from build123d import *

# Parameters (mm, degrees)
F0_W      = 25.4
F0_H      = 25.4
F1_DEPTH  = 25.4
F8_DEPTH  = 1.5875
F2_W      = 5.08
F2_H      = 17.78
F9_DEPTH  = 1.5875
F10_DEPTH = 1.5875
F11_DEPTH = 1.5875
F12_DEPTH = 1.5875
F13_DEPTH = 1.5875
F14_R     = 0.762


with BuildPart() as f1:
    # F0 (on Top) → F1 (new body)
    with BuildSketch(Plane.XY):
        Rectangle(F0_W, F0_H)
    extrude(amount=F1_DEPTH)

    # F7 (on face) → F8 (cut)
    with BuildSketch(Plane(origin=(-12.7, 0, 0), x_dir=(0, -1, 0), z_dir=(-1, 0, 0))):
        Polygon((-4.9953212532, 7.685226252), (-1.1170259365, 7.685226252), (-1.1170259365, 12.5987064093), (1.0614689121, 12.5987064093), (1.0614689121, 7.7727064093), (5.1815596911, 7.7727064093), (5.1815596911, 17.5121865667), (1.0614689121, 17.5121865667), (-1.1170259365, 17.5121865667), (-4.9953212532, 17.5121865667), align=None)
    extrude(amount=-F8_DEPTH, mode=Mode.SUBTRACT)

    # F2 (on face) → F9 (cut)
    with BuildSketch(Plane.XZ.offset(12.7)):
        with Locations((0, 12.7)):
            Rectangle(F2_W, F2_H)
    extrude(amount=-F9_DEPTH, mode=Mode.SUBTRACT)

    # F6 (on face) → F10 (cut)
    with BuildSketch(Plane.YZ.offset(12.7)):
        Polygon((0, 7.3222619789), (4.6011506993, 7.3222619789), (4.6011506993, 12.4022619789), (4.6011506993, 13.6722619789), (-2.54, 13.6722619789), (-2.54, 16.7535761464), (4.6011506993, 16.7535761464), (4.6011506993, 18.0235761464), (-2.54, 18.0235761464), (-3.81, 18.0235761464), (-3.81, 7.3222619789), (-2.54, 7.3222619789), (-2.54, 12.4022619789), (0, 12.4022619789), align=None)
    extrude(amount=-F10_DEPTH, mode=Mode.SUBTRACT)

    # F4 (on face) → F11 (cut)
    with BuildSketch(Plane(origin=(0, 12.7, 0), x_dir=(-1, 0, 0), z_dir=(0, 1, 0))):
        Polygon((6.35, 7.737770211), (6.35, 12.7), (-3.81, 12.7), (-3.81, 21.59), (-6.35, 21.59), (-6.35, 12.7), (-6.35, 7.737770211), align=None)
    extrude(amount=-F11_DEPTH, mode=Mode.SUBTRACT)

    # F3 (on face) → F12 (cut)
    with BuildSketch(Plane.XY.offset(25.4)):
        Polygon((-6.9272688269, 1.905), (-6.9272688269, -1.905), (3.1172688269, -1.905), (3.1172688269, -8.255), (6.9272688269, -8.255), (6.9272688269, -1.905), (6.9272688269, 1.905), (-3.1172688269, 1.905), (-3.1172688269, 8.255), (-6.9272688269, 8.255), align=None)
    extrude(amount=-F12_DEPTH, mode=Mode.SUBTRACT)

    # F5 (on face) → F13 (cut)
    with BuildSketch(Plane(origin=(0, 0, 0), x_dir=(1, 0, 0), z_dir=(0, 0, -1))):
        Polygon((-4.6181826849, 6.1575769132), (-4.6181826849, 1.0775769132), (4.6181826849, 1.0775769132), (4.6181826849, -1.0775769132), (-4.6181826849, -1.0775769132), (-4.6181826849, -6.1575769132), (4.6181826849, -6.1575769132), (7.8201234426, -6.1575769132), (7.8201234426, 6.1575769132), (4.6181826849, 6.1575769132), align=None)
    extrude(amount=-F13_DEPTH, mode=Mode.SUBTRACT)

    # F14
    f14_edges = [f1.edges().sort_by_distance(p)[0] for p in [
        (0, -12.7, 25.4),
        (-12.7, 0, 25.4),
        (12.7, 0, 25.4),
        (0, 12.7, 25.4),
        (-1.905, -1.905, 25.4),
        (3.117269, -5.08, 25.4),
        (5.022269, -8.255, 25.4),
        (6.927269, -3.175, 25.4),
        (1.905, 1.905, 25.4),
        (-3.117269, 5.08, 25.4),
        (-5.022269, 8.255, 25.4),
        (-6.927269, 3.175, 25.4),
        (-12.7, -12.7, 12.7),
        (0, -12.7, 0),
        (12.7, -12.7, 12.7),
        (-2.54, -12.7, 12.7),
        (0, -12.7, 21.59),
        (2.54, -12.7, 12.7),
        (0, -12.7, 3.81),
        (12.7, 0, 0),
        (12.7, 12.7, 12.7),
        (12.7, 0, 9.862262),
        (12.7, -1.27, 12.402262),
        (12.7, -2.54, 9.862262),
        (12.7, -3.175, 7.322262),
        (12.7, -3.81, 12.672919),
        (12.7, 0.395575, 18.023576),
        (12.7, 4.601151, 17.388576),
        (12.7, 1.030575, 16.753576),
        (12.7, -2.54, 15.212919),
        (12.7, 1.030575, 13.672262),
        (12.7, 4.601151, 10.497262),
        (12.7, 2.300575, 7.322262),
        (0, 12.7, 0),
        (-12.7, 12.7, 12.7),
        (0, 12.7, 7.73777),
        (6.35, 12.7, 14.663885),
        (5.08, 12.7, 21.59),
        (3.81, 12.7, 17.145),
        (-1.27, 12.7, 12.7),
        (-6.35, 12.7, 10.218885),
        (-12.7, 0, 0),
        (-12.7, -0.093119, 17.512187),
        (-12.7, -5.18156, 12.642446),
        (-12.7, -3.121514, 7.772706),
        (-12.7, -1.061469, 10.185706),
        (-12.7, 0.027779, 12.598706),
        (-12.7, 1.117026, 10.141966),
        (-12.7, 3.056174, 7.685226),
        (-12.7, 4.995321, 12.598706),
        (1.60097, 6.157577, 0),
        (-4.618183, 3.617577, 0),
        (0, 1.077577, 0),
        (4.618183, 0, 0),
        (0, -1.077577, 0),
        (-4.618183, -3.617577, 0),
        (1.60097, -6.157577, 0),
        (7.820123, 0, 0),
    ]]
    fillet(f14_edges, radius=F14_R)


solid = f1.part
Design review of the part built by this model. Coordinates are the model's own, in mm. A direction names the side the tool comes from. Give positions to 0.01 mm unless a question says otherwise; leave off trailing zeros. Loops run counter-clockwise (first coordinate to the right, second up) from the corner with the lowest first, then second, coordinate; pieces in that order, holes last. Notation, with made-up numbers: (-18.5, -32.5) - (23.5, -32.5) arc R24 cw to (23.5, -6.5) - close; hole circle Ø10 at (-33.75, 70.5). An arc over 180 degrees is marked (long way). Write item = value, one per line.
1) To check wall thickness, follow line 1 (X direction, y = -2.5, z = 1); line 2 (X direction, y = 11.5, z = 10.75); line 3 (Y direction, x = 6, z = 19). State the ranges of each line that lie inside material, in increasing order.
Result sheet:
line_1 = -12.7 to -4.62, 7.82 to 12.7
line_2 = -12.7 to -6.35, 6.35 to 12.7
line_3 = -12.7 to 11.11
2) Clearance check with a flat-ended pin moving along its axis: pin 1 Ø5 at (y, z) = (3.5, 11) entering from +X. State where the tip first meets the part, or that it passes through.
Result sheet:
pin_1 = 12.7
3) Draft analysis for pull direction Z (two halves, no side actions). For faces 1 (the face through (0, 3, 25.4)), 2 (the face through (5, -8.255, 24)), 3 (the face through (0.1, 11.5, 7.738)), state which applies: +Z half, -Z half, draft (parallel to the pull), parting line (faces both ways), or undercut.
Result sheet:
face_1 = +Z half
face_2 = draft
face_3 = undercut
4) Take a section at B-B on z = 19.75. State the section outline as (x, y) points, and give its area (3 significant figures).
Result sheet:
outline = (-12.7, -11.94) arc R0.76 ccw to (-11.94, -12.7) - (-3.3, -12.7) arc R0.76 ccw to (-2.54, -11.94) - (-2.54, -11.11) - (2.54, -11.11) - (2.54, -11.94) arc R0.76 ccw to (3.3, -12.7) - (11.94, -12.7) arc R0.76 ccw to (12.7, -11.94) - (12.7, 11.94) arc R0.76 ccw to (11.94, 12.7) - (7.11, 12.7) arc R0.76 ccw to (6.35, 11.94) - (6.35, 11.11) - (3.81, 11.11) - (3.81, 11.94) arc R0.76 ccw to (3.05, 12.7) - (-11.94, 12.7) arc R0.76 ccw to (-12.7, 11.94) - close
area = 632 mm2
5) Tool access review of faces 4 (the face through (-11.5, -1.061, 10.2)), 5 (the face through (-1.3, 11.5, 12.7)), 6 (the face through (7.82, 0, 1)): name each direction out of +Z, -Z, +X, -X, +Y, -Y from which nothing blocks a thin tool from reaching the whole face with its end or side.
Result sheet:
face_4 = -X
face_5 = +Y
face_6 = -Z
